Read the model definition and answer for the solid it produces. Units are mm, in the model's axes. A direction names the side the tool comes from. Coordinates: 2 decimals unless noted, no trailing zeros. Write each loop counter-clockwise with the first axis right and the second up, starting at its lowest first coordinate (ties: lowest second). Pieces come first, ordered by that corner, then holes. Notation, with made-up numbers: (-25, 65) - (30, 65) arc R10 cw to (30, 69) - close; hole circle Ø8 at (-22.5, -21.75). An arc over 180 degrees is marked (long way). Return JSON: item names as keys, results as strings.
```python
from build123d import *

# Parameters (mm, degrees)
F0_R     = 2.5
F1_DEPTH = 3


# Not quite as in the source:
# - a fillet or chamfer that OpenCascade refuses, or shapes differently, is made with other operations: its cross-section is extruded or revolved along the edge and cut away or added


with BuildPart() as f1:
    # F0 (on Front) → F1 (new body)
    with BuildSketch(Plane.XZ):
        with BuildLine():
            Line((40.1844298095, -16.8644712743), (40.1844298095, 13.8644712743))
            ThreePointArc((40.1844298095, 13.8644712743), (40.4994101244, 17.4000051803), (41.4344298095, 20.8241767279))
            ThreePointArc((41.4344298095, 20.8241767279), (35.0877662109, 35.9525016382), (19.5764143341, 30.6098135152))
            ThreePointArc((19.5764143341, 30.6098135152), (12.2164228481, 22.827751719), (1.8963885419, 19.9595027072))
            Line((1.8963885419, 19.9595027072), (-30, 19.9595027072))
            ThreePointArc((-30, 19.9595027072), (-37.0710678119, 17.030570519), (-40, 9.9595027072))
            Line((-40, 9.9595027072), (-40, -10.0404972928))
            ThreePointArc((-40, -10.0404972928), (-37.0710678119, -17.1115651047), (-30, -20.0404972928))
            Line((-30, -20.0404972928), (0.5360500065, -20.0404972928))
            ThreePointArc((0.5360500065, -20.0404972928), (11.7050648207, -23.4497436005), (19.0662873833, -32.5151864848))
            ThreePointArc((19.0662873833, -32.5151864848), (34.5304347857, -39.18535832), (41.4344298095, -23.8241767279))
            ThreePointArc((41.4344298095, -23.8241767279), (40.4994101244, -20.4000051803), (40.1844298095, -16.8644712743))
        make_face()
        with BuildLine():
            ThreePointArc((-30, -7.5404972928), (-28.232233047, -8.2727303399), (-27.5, -10.0404972928))
            ThreePointArc((-27.5, -10.0404972928), (-31.767766953, -11.8082642458), (-30, -7.5404972928))
        make_face(mode=Mode.SUBTRACT)
        with Locations((30.1844298095, -28)):
            Circle(F0_R, mode=Mode.SUBTRACT)
        with Locations((30.1844298095, -10)):
            Circle(F0_R, mode=Mode.SUBTRACT)
        with BuildLine():
            ThreePointArc((-26.5, 9.9595027072), (-27.5251262658, 7.484628973), (-30, 6.4595027072))
            ThreePointArc((-30, 6.4595027072), (-32.4748737342, 12.4343764413), (-26.5, 9.9595027072))
        make_face(mode=Mode.SUBTRACT)
        with Locations((30.1844298095, 10)):
            Circle(F0_R, mode=Mode.SUBTRACT)
        with Locations((30.1844298095, 25)):
            Circle(F0_R, mode=Mode.SUBTRACT)
    extrude(amount=F1_DEPTH)

    # F2: chamfer of 3.5 on 3 edges, made by hand

    # F2_s1 → F2_t2 (revolve, cut)
    with BuildSketch(Plane.YZ.offset(-30)):
        Polygon((-3, -4.0404972928), (0.5, -7.5404972928), (-3, -7.5404972928), align=None)
    revolve(axis=Axis((-30, -3, -10.0404972928), (0, -1, 0)), mode=Mode.SUBTRACT)

    # F2_s3 → F2_t4 (revolve, cut)
    with BuildSketch(Plane.XY.offset(-10)):
        Polygon((36.1844298095, -3), (32.6844298095, 0.5), (32.6844298095, -3), align=None)
    revolve(axis=Axis((30.1844298095, -3, -10), (0, -1, 0)), mode=Mode.SUBTRACT)

    # F2_s5 → F2_t6 (revolve, cut)
    with BuildSketch(Plane.XY.offset(10)):
        Polygon((36.1844298095, -3), (32.6844298095, 0.5), (32.6844298095, -3), align=None)
    revolve(axis=Axis((30.1844298095, -3, 10), (0, -1, 0)), mode=Mode.SUBTRACT)


solid = f1.part
```
(1) A cutting plane is placed at A-A (z = 26). Determine the outline of the cut face in (x, y), and give its area (3 significant figures).
Answer:
{"outline": "(16.22, -3) - (27.89, -3) - (27.89, 0) - (16.22, 0) - close; (32.48, -3) - (42.14, -3) - (42.14, 0) - (32.48, 0) - close", "area": "64.0 mm²"}
(2) A cutting plane is placed at D-D (z = -27). Determine the outline of the cut face in (x, y), and give its area (3 significant figures).
Answer:
{"outline": "(15.7, -3) - (27.89, -3) - (27.89, 0) - (15.7, 0) - close; (32.48, -3) - (42.14, -3) - (42.14, 0) - (32.48, 0) - close", "area": "65.6 mm²"}
(3) Straight lines are drawn through the part: line 1 (X direction, y = -2.4, z = 9); line 2 (Z direction, x = 27, y = -2.55); line 3 (Z direction, x = -30, y = -0.4). For each, find the intervals that lie inside material, in ascending order. Write a range as from..to.
Answer:
{"line 1": "-40..-33.37, -26.63..24.88, 35.49..40.18", "line 2": "-39.57..-14.55, -5.45..5.45, 14.55..36.57", "line 3": "-20.04..-13.44, -6.64..6.46, 13.46..19.96"}
(4) Flat-ended cylindrical pins translate along their axes: P1, Ø1, axis at y = -1.5, z = 20.5, coming from the +X side; P2, Ø8, axis at x = 30.18, z = 25, coming from the +Y side. Find the tip coordinate at first contact, or state that the pin passes through.
Answer:
{"P1": "x = 41.5", "P2": "y = 0"}
(5) Determine the mould class of faces 5 (the face through (32.57, -1.48, 25.75)), 6 (the face through (40.184, -1, -2)), 7 (the face through (10, -3, -1)) for opening direction X: +X half, -X half, draft (parallel to the pull), parting line (faces both ways), or undercut.
Answer:
{"face 5": "undercut", "face 6": "+X half", "face 7": "draft"}
(6) A cutting plane is placed at C-C (x = -21.5). Determine the outline of the cut face in (y, z).
Answer:
{"outline": "(-3, -20.04) - (0, -20.04) - (0, 19.96) - (-3, 19.96) - close"}
(7) Which of the six approach directions +Z, -Z, +X, -X, +Y, -Y give full straight-line access (tool end or side, diameter ignored) to faces 1 (the face through (40.5, -1.5, -20.4)), 2 (the face through (-14, -1, 19.96)), 3 (the face through (-15, -1, -20.04)), 4 (the face through (10, 0, -1))?
Answer:
{"face 1": "+X, +Y, -Y", "face 2": "+Z, -X, +Y, -Y", "face 3": "-Z, -X, +Y, -Y", "face 4": "+Z, -Z, +X, -X, +Y"}
(8) A cutting plane is placed at B-B (y = -0.7). Determine the outline of the cut face in (x, z), and give its area (3 significant figures).
Answer:
{"outline": "(-40, -10.04) arc R10 ccw to (-30, -20.04) - (0.54, -20.04) arc R20 cw to (19.07, -32.52) arc R12 ccw to (41.43, -23.82) arc R20 cw to (40.18, -16.86) - (40.18, 13.86) arc R20 cw to (41.43, 20.82) arc R12 ccw to (19.58, 30.61) arc R20 cw to (1.9, 19.96) - (-30, 19.96) arc R10 ccw to (-40, 9.96) - close; hole circle Ø7.4 at (-30, -10.04); hole circle Ø7 at (-30, 9.96); hole circle Ø7.4 at (30.18, -10); hole circle Ø7.4 at (30.18, 10); hole circle Ø5 at (30.18, -28); hole circle Ø5 at (30.18, 25)", "area": "3,810 mm²"}
